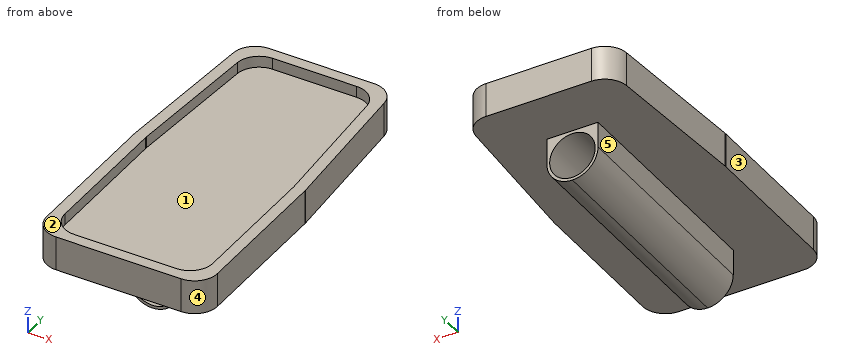
from build123d import *

# Parameters (mm, degrees)
F1_DEPTH    = 30
F2_DEPTH    = 20
F3_T1_DEPTH = 10
F3_T3_DEPTH = 11.6648189186
F3_T5_DEPTH = 130
F3_T7_DEPTH = 123.5553091892
F3_T9_DEPTH = 33.3296378373
F5_W        = 45
F5_H        = 200
F6_DEPTH    = 45
F7_R        = 20
F8_DEPTH    = 200
F9_R        = 22.49999


# Not quite as in the source:
# - a fillet or chamfer that OpenCascade refuses, or shapes differently, is made with other operations: its cross-section is extruded or revolved along the edge and cut away or added
# - two fillets or chamfers of one size are made in one step
# - a fillet or chamfer is up to 0.001 mm smaller than in the source, because OpenCascade refuses the exact size


with BuildPart() as f1:
    # F0 (on Top) → F1 (new body)
    with BuildSketch(Plane.XY):
        Polygon((65, 150), (-65, 150), (-75, 0), (-75, -150), (75, -150), (75, 0), align=None)
        Polygon((-65, 0), (-55.6666666667, 140), (55.6666666667, 140), (65, 0), (65, -140), (-65, -140), align=None, mode=Mode.SUBTRACT)
    extrude(amount=F1_DEPTH)

    # F0 (on Top) → F2 (join)
    with BuildSketch(Plane.XY):
        Polygon((55.6666666667, 140), (-55.6666666667, 140), (-65, 0), (-65, -140), (65, -140), (65, 0), align=None)
    extrude(amount=F2_DEPTH)

    # F3: fillet of radius 20 on 12 edges, made by hand

    # F3_s2 → F3_t1 (join)
    with BuildSketch(Plane.XY.offset(20)):
        with BuildLine():
            ThreePointArc((-56.911307986, 121.3303802105), (-50.6192865397, 134.6049238993), (-36.9556048288, 140))
            Line((-36.9556048288, 140), (-55.6666666667, 140))
            Line((-55.6666666667, 140), (-56.911307986, 121.3303802105))
        make_face()
        with BuildLine():
            ThreePointArc((36.9556048288, 140), (50.6192865397, 134.6049238993), (56.911307986, 121.3303802105))
            Line((56.911307986, 121.3303802105), (55.6666666667, 140))
            Line((55.6666666667, 140), (36.9556048288, 140))
        make_face()
        with BuildLine():
            ThreePointArc((65, -120), (59.1421356237, -134.1421356237), (45, -140))
            Line((45, -140), (65, -140))
            Line((65, -140), (65, -120))
        make_face()
        with BuildLine():
            ThreePointArc((-45, -140), (-59.1421356237, -134.1421356237), (-65, -120))
            Line((-65, -120), (-65, -140))
            Line((-65, -140), (-45, -140))
        make_face()
    extrude(amount=F3_T1_DEPTH)

    # F3_s4 → F3_t3 (join)
    with BuildSketch(Plane.XY.offset(18.3351810814)):
        with BuildLine():
            ThreePointArc((-64.9557031571, 0.664452643), (-64.9889227216, -0.0003688333), (-65, -0.6659275675))
            Line((-65, -0.6659275675), (-65, 0))
            Line((-65, 0), (-64.9557031571, 0.664452643))
        make_face()
        with BuildLine():
            ThreePointArc((64.9557031571, 0.664452643), (64.9889227216, -0.0003688333), (65, -0.6659275675))
            Line((65, -0.6659275675), (65, 0))
            Line((65, 0), (64.9557031571, 0.664452643))
        make_face()
    extrude(amount=F3_T3_DEPTH)

    # F3_s6 → F3_t5 (cut)
    with BuildSketch(Plane.XY.offset(-50)):
        with BuildLine():
            ThreePointArc((75, -130), (69.1421356237, -144.1421356237), (55, -150))
            Line((55, -150), (75, -150))
            Line((75, -150), (75, -130))
        make_face()
        with BuildLine():
            ThreePointArc((-75, -130), (-69.1421356237, -144.1421356237), (-55, -150))
            Line((-55, -150), (-75, -150))
            Line((-75, -150), (-75, -130))
        make_face()
    extrude(amount=F3_T5_DEPTH, mode=Mode.SUBTRACT)

    # F3_s8 → F3_t7 (cut)
    with BuildSketch(Plane.XY.offset(-46.7776545946)):
        with BuildLine():
            ThreePointArc((46.2889381622, 150), (59.952619873, 144.6049238993), (66.2446413193, 131.3303802105))
            Line((66.2446413193, 131.3303802105), (65, 150))
            Line((65, 150), (46.2889381622, 150))
        make_face()
        with BuildLine():
            ThreePointArc((-46.2889381622, 150), (-59.952619873, 144.6049238993), (-66.2446413193, 131.3303802105))
            Line((-66.2446413193, 131.3303802105), (-65, 150))
            Line((-65, 150), (-46.2889381622, 150))
        make_face()
    extrude(amount=F3_T7_DEPTH, mode=Mode.SUBTRACT)

    # F3_s10 → F3_t9 (cut)
    with BuildSketch(Plane.XY.offset(-1.6648189186)):
        with BuildLine():
            ThreePointArc((74.9557031571, 0.664452643), (74.9889227216, -0.0003688333), (75, -0.6659275675))
            Line((75, -0.6659275675), (75, 0))
            Line((75, 0), (74.9557031571, 0.664452643))
        make_face()
        with BuildLine():
            ThreePointArc((-74.9557031571, 0.664452643), (-74.9889227216, -0.0003688333), (-75, -0.6659275675))
            Line((-75, -0.6659275675), (-75, 0))
            Line((-75, 0), (-74.9557031571, 0.664452643))
        make_face()
    extrude(amount=F3_T9_DEPTH, mode=Mode.SUBTRACT)

    # F5 (on face) → F6 (join)
    with BuildSketch(Plane.XY):
        Rectangle(F5_W, F5_H)
    extrude(amount=-F6_DEPTH)

    # F7 (on face) → F8 (cut, through all)
    with BuildSketch(Plane.XZ.offset(100)):
        with Locations((0, -22.5)):
            Circle(F7_R)
    extrude(amount=-F8_DEPTH, mode=Mode.SUBTRACT)

    # F9 (radius 22.5 in the source; OpenCascade refuses exactly that, so slightly less here)
    f9_edges = [f1.edges().sort_by_distance(p)[0] for p in [
        (-22.5, 0, -45),
        (22.5, 0, -45),
    ]]
    fillet(f9_edges, radius=F9_R)


solid = f1.part
Read the model definition and answer for the solid it produces. Units are mm, in the model's axes. Face numbers are marked on the shaded views. A direction names the side the tool comes from. Round coordinates to 2 decimals unless told otherwise and drop trailing zeros. Write each loop counter-clockwise with the first axis right and the second up, starting at its lowest first coordinate (ties: lowest second). Pieces come first, ordered by that corner, then holes. Notation, with made-up numbers: M 11.5,1 L 17.5,1 A24 ccw 17.5,16 Z; hole C -29,-8 d11. An arc over 180 degrees is marked long. Use a Markdown table: item, result.
1) The part is cut by section A-A (z = -9). Write down the section's boundary in (x, y).
Answers follow:
| item | result |
|---|---|
| outline | M -22.5,-100 L -14.76,-100 L -14.76,100 L -22.5,100 Z; M 14.76,-100 L 22.5,-100 L 22.5,100 L 14.76,100 Z |
2) For a pull along X with two mould halves and no side action, classify the marked faces 1, 2 and 3 as pulls with the +X half, pulls with the -X half, needs draft (parallel to the pull), parting line crosses it, or undercut.
Answers follow:
| item | result |
|---|---|
| face 1 | undercut |
| face 2 | needs draft |
| face 3 | pulls with the -X half |
3) Flat-ended cylindrical pins translate along their axes: pin 1 (12 mm diameter, centred on y = 104.5, z = -33, fed in from -X); pin 2 (12 mm diameter, centred on x = -46, y = -32, fed in from +Z); pin 3 (1.5 mm diameter, centred on x = -59.5, z = 3.5, fed in from +Y). Find the tip coordinate at first contact, or state that the pin passes through.
Answers follow:
| item | result |
|---|---|
| pin 1 | stops at x = -21.53 |
| pin 2 | stops at z = 20 |
| pin 3 | stops at y = 145.64 |
4) A tool of negligible diameter and unlimited length cuts with its end or side. For the marked faces 4 and 5, from which of +Z, -Z, +X, -X, +Y, -Y can it reach the whole face along a straight path? Write none if from no direction.
Answers follow:
| item | result |
|---|---|
| face 4 | +Z, -Z, +X, -Y |
| face 5 | -Z, -X, +Y, -Y |
5) The part is cut by section C-C (z = 12). Write down the section's boundary in (x, y), plus the area to 3 significant figures.
Answers follow:
| item | result |
|---|---|
| outline | M -75,-130 A20 ccw -55,-150 L 55,-150 A20 ccw 75,-130 L 75,-0.67 A20 ccw 74.96,0.66 L 66.24,131.33 A20 ccw 46.29,150 L -46.29,150 A20 ccw -66.24,131.33 L -74.96,0.66 A20 ccw -75,-0.67 Z |
| area | 43,200 mm2 |
6) Straight lines are drawn through the part: line 1 along X through (y, z) = (-44, -22); line 2 along Y through (x, z) = (-1, 27); line 3 along Z through (x, y) = (-46.5, -109). For each, find the intervals that lie inside material, in ascending order. Write a range as [from, to].
Answers follow:
| item | result |
|---|---|
| line 1 | x = [-22.5, -19.99], [19.99, 22.5] |
| line 2 | y = [-150, -140], [140, 150] |
| line 3 | z = [0, 20] |
7) The part is cut by section D-D (x = -12.5). Write down the section's boundary in (y, z), plus the area to 3 significant figures.
Answers follow:
| item | result |
|---|---|
| outline | M -150,0 L -100,0 L -100,-6.89 L 100,-6.89 L 100,0 L 150,0 L 150,30 L 140,30 L 140,20 L -140,20 L -140,30 L -150,30 Z; M -100,-41.21 L 100,-41.21 L 100,-38.11 L -100,-38.11 Z |
| area | 8,200 mm2 |
